from build123d import *

# Parameters (mm, degrees)
SKETCH_1_W             = 135
SKETCH_1_H             = 70
EXTRUDE_1_DEPTH        = 45
SKETCH_2_W             = 133
SKETCH_2_H             = 68
CUT_EXTRUDE_1_DEPTH    = 10
SKETCH_4_W             = 131
SKETCH_4_H             = 66
CUT_EXTRUDE_3_DEPTH    = 33
FILLET_3_R             = 20
SKETCH_5_W             = 10
SKETCH_5_H             = 1.4
EXTRUDE_2_DEPTH        = 0.7
FILLET_5_R             = 0.7
FILLET_5_OF_MIRROR_2_R = 0.7
SKETCH_6_W             = 10
SKETCH_6_H             = 1.4
EXTRUDE_3_DEPTH        = 0.7
FILLET_6_R             = 0.7
FILLET_6_OF_MIRROR_3_R = 0.7


with BuildPart() as part:
    # 草图1 → 凸台-拉伸1 (new body)
    with BuildSketch(Plane(origin=(0, 0, 0), x_dir=(1, 0, 0), z_dir=(0, 1, 0))):
        Rectangle(SKETCH_1_W, SKETCH_1_H)
    extrude(amount=EXTRUDE_1_DEPTH)

    # 草图2 → 切除-拉伸1 (cut)
    with BuildSketch(Plane(origin=(0, 45, 0), x_dir=(1, 0, 0), z_dir=(0, 1, 0))):
        Rectangle(SKETCH_2_W, SKETCH_2_H)
    extrude(amount=-CUT_EXTRUDE_1_DEPTH, mode=Mode.SUBTRACT)

    # 草图4 → 切除-拉伸3 (cut)
    with BuildSketch(Plane(origin=(0, 35, 0), x_dir=(1, 0, 0), z_dir=(0, 1, 0))):
        Rectangle(SKETCH_4_W, SKETCH_4_H)
    extrude(amount=-CUT_EXTRUDE_3_DEPTH, mode=Mode.SUBTRACT)

    # 圆角3
    fillet_3_edges = [part.edges().sort_by_distance(p)[0] for p in [
        (-66.5, 40, -34),
        (66.5, 40, -34),
        (66.5, 40, 34),
        (-66.5, 40, 34),
        (65.5, 18.5, -33),
        (-65.5, 18.5, -33),
        (-65.5, 18.5, 33),
        (65.5, 18.5, 33),
        (-67.5, 22.5, 35),
        (67.5, 22.5, 35),
        (67.5, 22.5, -35),
        (-67.5, 22.5, -35),
    ]]
    fillet(fillet_3_edges, radius=FILLET_3_R)

    # 草图5 → 凸台-拉伸2 (add)
    with BuildSketch(Plane.XY.offset(-34)):
        with Locations((0, 40)):
            Rectangle(SKETCH_5_W, SKETCH_5_H)
    extrude_2 = extrude(amount=EXTRUDE_2_DEPTH)

    # 圆角5
    fillet_5_edges = [part.edges().sort_by_distance(p)[0] for p in [
        (5, 40, -33.3),
        (-5, 40, -33.3),
        (0, 39.3, -33.3),
        (0, 40.7, -33.3),
    ]]
    fillet(fillet_5_edges, radius=FILLET_5_R - 0.0001)  # a hair under: the kernel refuses the full size

    # 镜向2: 凸台-拉伸2 across plane
    add(extrude_2.mirror(Plane.XY))

    # 圆角5 of 镜向2
    fillet_5_of_mirror_2_edges = [part.edges().sort_by_distance(p)[0] for p in [
        (5, 40, 33.3),
        (-5, 40, 33.3),
        (0, 39.3, 33.3),
        (0, 40.7, 33.3),
    ]]
    fillet(fillet_5_of_mirror_2_edges, radius=FILLET_5_OF_MIRROR_2_R - 0.0001)  # a hair under: the kernel refuses the full size

    # 草图6 → 凸台-拉伸3 (add)
    with BuildSketch(Plane(origin=(-66.5, 0, 0), x_dir=(0, 0, -1), z_dir=(1, 0, 0))):
        with Locations((0, 40)):
            Rectangle(SKETCH_6_W, SKETCH_6_H)
    extrude_3 = extrude(amount=EXTRUDE_3_DEPTH)

    # 圆角6
    fillet_6_edges = [part.edges().sort_by_distance(p)[0] for p in [
        (-65.8, 40, -5),
        (-65.8, 40, 5),
        (-65.8, 39.3, 0),
        (-65.8, 40.7, 0),
    ]]
    fillet(fillet_6_edges, radius=FILLET_6_R - 0.0001)  # a hair under: the kernel refuses the full size

    # 镜向3: 凸台-拉伸3 across plane
    add(extrude_3.mirror(Plane(origin=(0, 0, 0), x_dir=(0, 0, 1), z_dir=(1, 0, 0))))

    # 圆角6 of 镜向3
    fillet_6_of_mirror_3_edges = [part.edges().sort_by_distance(p)[0] for p in [
        (65.8, 40, -5),
        (65.8, 40, 5),
        (65.8, 39.3, 0),
        (65.8, 40.7, 0),
    ]]
    fillet(fillet_6_of_mirror_3_edges, radius=FILLET_6_OF_MIRROR_3_R - 0.0001)  # a hair under: the kernel refuses the full size


solid = part.part
Model file for the job. Use its own axes, mm. A direction names the side the tool comes from. Give positions to 0.01 mm unless a question says otherwise; leave off trailing zeros. Order: outer loops, then holes, each group sorted by start corner. A loop starts at its lowest first (then second) coordinate and runs counter-clockwise, first axis right, second up. Notation, with made-up numbers: (-12.5, 22.25) - (23.5, 22.25) arc R10 cw to (23.5, 31.25) - close; hole circle Ø1 at (-30, -12.5). An arc over 180 degrees is marked (long way). Write item = value, one per line. Start each with the question number.
1. Drop a flat-ended pin along its axis: P1, Ø10, axis at x = 27, z = 4.5, coming from the +Y side. Give the stop position or say it passes through.
2. Probe line 1 along Z through (x, y) = (-9.5, 24.5); line 2 along X through (y, z) = (27, -10.5); line 3 along Z through (x, y) = (-25, 38.5). List the from-to ranges inside material, lowest first.
3. Which spindle directions (+Z, -Z, +X, -X, +Y, -Y) get a long thin tool onto all of the face, cutting with end or side? Do faces 5 (the flat face through (-1, 0, 0)), 6 (the flat face through (-66.5, 41, 0)), 7 (the cylindrical face through (59.797, 18.269, -26.986)). Say none if no direction does.
4. Two-plate mould, pull along Z, no slides. Class faces 1 (the cylindrical face through (61.486, 22.815, 29.297)), 2 (the flat face through (-50, 35, 33)), 3 (the cylindrical face through (60.486, 39.93, 28.297)), 4 (the cylindrical face through (-61.797, 22.815, -28.986)): pulls with the +Z half, pulls with the -Z half, needs draft (parallel to the pull), parting line crosses it, or undercut.
5. Cut at A-A, the plane y = 42. List the corners of the cut face in (x, z).
6. Cut at C-C, the plane x = -15. List the corners of the cut face in (y, z).
7. Cut at D-D, the plane y = 16. List the corners of the cut face in (x, z).
Taken from the geometry:
q1.P1 = 2
q2.line_1 = -35 to -33, 33 to 35
q2.line_2 = -67.5 to -65.5, 65.5 to 67.5
q2.line_3 = -35 to -34, 34 to 35
q3.face_5 = +Z, -Z, +X, -X, -Y
q3.face_6 = none
q3.face_7 = +Y
q4.face_1 = pulls with the +Z half
q4.face_2 = undercut
q4.face_3 = undercut
q4.face_4 = pulls with the -Z half
q5.outline = (-67.5, -15) arc R20 ccw to (-47.5, -35) - (47.5, -35) arc R20 ccw to (67.5, -15) - (67.5, 15) arc R20 ccw to (47.5, 35) - (-47.5, 35) arc R20 ccw to (-67.5, 15) - close; hole (-66.5, -14) arc R20 ccw to (-46.5, -34) - (46.5, -34) arc R20 ccw to (66.5, -14) - (66.5, 14) arc R20 ccw to (46.5, 34) - (-46.5, 34) arc R20 ccw to (-66.5, 14) - close
q6.outline = (0, -35) - (45, -35) - (45, -34) - (35, -34) - (35, -33) - (2, -33) - (2, 33) - (35, 33) - (35, 34) - (45, 34) - (45, 35) - (0, 35) - close
q7.outline = (-67.5, -15) arc R20 ccw to (-47.5, -35) - (47.5, -35) arc R20 ccw to (67.5, -15) - (67.5, 15) arc R20 ccw to (47.5, 35) - (-47.5, 35) arc R20 ccw to (-67.5, 15) - close; hole (-65.5, -13) arc R20 ccw to (-45.5, -33) - (45.5, -33) arc R20 ccw to (65.5, -13) - (65.5, 13) arc R20 ccw to (45.5, 33) - (-45.5, 33) arc R20 ccw to (-65.5, 13) - close
